```python
from build123d import *

# Parameters (mm, degrees)
F0_W      = 50.8
F0_H      = 50.8
F1_DEPTH  = 50.8
F2_R      = 9
F3_DEPTH  = 407.416
F4_W      = 60.1204171121
F4_H      = 25.4
F5_DEPTH  = 338.582
F6_R      = 5.08
F7_DEPTH  = 5.08
F8_R      = 2.159
F9_DEPTH  = 25.4
F10_R     = 1.5494
F11_DEPTH = 25.4
F12_R     = 1.5494
F12_R_2   = 2.159
F13_DEPTH = 25.4
F14_R     = 5.08
F15_DEPTH = 5.08
F19_DEPTH = 72.39
F22_R     = 12.7


with BuildPart() as f1:
    # F0 (on Top) → F1 (new body)
    with BuildSketch(Plane.XY):
        Rectangle(F0_W, F0_H)
    extrude(amount=F1_DEPTH)

    # F2 (on face) → F3 (cut)
    with BuildSketch(Plane(origin=(0, 0, 0), x_dir=(1, 0, 0), z_dir=(0, 0, -1))):
        Circle(F2_R)
    extrude(amount=-F3_DEPTH, mode=Mode.SUBTRACT)

    # F4 (on face) → F5 (cut)
    with BuildSketch(Plane(origin=(0, 0, 0), x_dir=(1, 0, 0), z_dir=(0, 0, -1))):
        with Locations((4.6602085561, 12.7)):
            Rectangle(F4_W, F4_H)
    extrude(amount=-F5_DEPTH, mode=Mode.SUBTRACT)

    # F6 (on face) → F7 (cut)
    with BuildSketch(Plane.XZ):
        with Locations((-17.2, 25.4)):
            Circle(F6_R)
    extrude(amount=-F7_DEPTH, mode=Mode.SUBTRACT)

    # F8 (on face) → F9 (cut)
    with BuildSketch(Plane.XZ.offset(-5.08)):
        with Locations((-17.2, 25.4)):
            Circle(F8_R)
    extrude(amount=-F9_DEPTH, mode=Mode.SUBTRACT)

    # F10 (on face) → F11 (cut)
    with BuildSketch(Plane.XZ):
        with Locations((-17.2, 44.4713309407)):
            Circle(F10_R)
    extrude(amount=-F11_DEPTH, mode=Mode.SUBTRACT)

    # F12 (on face) → F13 (cut)
    with BuildSketch(Plane.XZ):
        with Locations((17.2, 44.4713309407)):
            Circle(F12_R)
        with Locations((17.2, 25.4)):
            Circle(F12_R_2)
    extrude(amount=-F13_DEPTH, mode=Mode.SUBTRACT)

    # F14 (on face) → F15 (cut)
    with BuildSketch(Plane.XZ):
        with Locations((17.2, 25.4)):
            Circle(F14_R)
    extrude(amount=-F15_DEPTH, mode=Mode.SUBTRACT)

    # F17: F1 across plane


with BuildPart() as f1_1:
    add(f1.part)
    add(f1.part.mirror(Plane(origin=(0, 13.6714489466, 25.4), x_dir=(1, 0, 0), z_dir=(0, 0, 1))), mode=Mode.INTERSECT)

    # F18 (on face) → F19 (cut)
    with BuildSketch(Plane(origin=(0, 0, 0), x_dir=(1, 0, 0), z_dir=(0, 0, -1))):
        Polygon((37.3146161437, -15.35), (0, -15.35), (-44.7141490877, -15.35), (-42.6479764283, -31.9298505783), (43.3826521039, -33.9571945369), align=None)
    extrude(amount=-F19_DEPTH, mode=Mode.SUBTRACT)

    # F22
    f22_edges = [f1_1.edges().sort_by_distance(p)[0] for p in [
        (25.4, 7.675, 50.8),
        (25.4, 7.675, 0),
        (-25.4, 7.675, 50.8),
        (-25.4, 7.675, 0),
    ]]
    fillet(f22_edges, radius=F22_R)


solid = f1_1.part
```
The model under review builds one solid part; all positions refer to its coordinate system, in mm. A direction names the side the tool comes from. Give positions to 0.01 mm unless a question says otherwise; leave off trailing zeros. Write each loop counter-clockwise with the first axis right and the second up, starting at its lowest first coordinate (ties: lowest second). Pieces come first, ordered by that corner, then holes. Notation, with made-up numbers: M 7.5,68 L 61.5,68 A11 cw 61.5,87 Z; hole C 4.5,58.25 d2. An arc over 180 degrees is marked long. Write each question's results on one line, items separated by ' | '. Start each with the question number.
1. We need section B-B (z = 25.4). Write out the cut boundary in (x, y).
2. Insertion check: pin 1 Ø5.5 at (x, z) = (-17.2, 25.4) entering from -Y; pin 2 Ø3 at (x, y) = (18, 11) entering from +Z; pin 3 Ø1.9 at (x, z) = (17.2, 44.47) entering from -Y. Each pin has a flat end and moves straight along its axis. Give the tip position at first contact, or say it passes through.
3. For probe 1 along Z at (x, y) = (-17.2, 3.95); probe 2 along Z at (x, y) = (-17.2, 8.75); probe 3 along X at (y, z) = (12.25, 44), list the stretches that pass through material, from the lowest coordinate up. Write a range as [from, to].
4. Mouldability with a two-part tool opening along X and no side actions: class faces 1 (the flat face through (25.4, 8, 25)), 2 (the cylindrical face through (16.86, 7.57, 7.84)), 3 (the flat face through (-0.2, 9.5, 0)) as released by +X, released by -X, zero draft, split by the parting line, or undercut.
5. We need section C-C (x = 17.2). Write out the cut boundary in (y, z), and give its area (3 significant figures).
6. For faces 4 (the cylindrical face through (0, 9, 25)), 5 (the cylindrical face through (-20.944, 2.504, 28.833)), list the 3-axis set-ups (+Z, -Z, +X, -X, +Y, -Y) from which the entire face can be reached by the end or side of a thin tool; tool diameter is ignored.
7. We need section A-A (y = 7.75). Write out the cut boundary in (x, z).
8. We need section D-D (y = 11.5). Write out the cut boundary in (x, z).
Results found:
1) outline: M -25.4,0 L -22.28,0 L -22.28,5.08 L -19.36,5.08 L -19.36,15.35 L -25.4,15.35 Z; M -15.04,5.08 L -12.12,5.08 L -12.12,0 L -9,0 A9 cw 9,0 L 12.12,0 L 12.12,5.08 L 15.04,5.08 L 15.04,15.35 L -15.04,15.35 Z; M 19.36,5.08 L 22.28,5.08 L 22.28,0 L 25.4,0 L 25.4,15.35 L 19.36,15.35 Z
2) pin 1: stops at y = 5.08 | pin 2: stops at z = 50.22 | pin 3: passes through
3) probe 1: z = [0.82, 4.78], [7.88, 20.32], [30.48, 42.92], [46.02, 49.98] | probe 2: z = [0.82, 4.78], [7.88, 23.24], [27.56, 42.92], [46.02, 49.98] | probe 3: x = [-23.95, -18.68], [-15.72, 15.72], [18.68, 23.95]
4) face 1: released by +X | face 2: undercut | face 3: zero draft
5) outline: M 0,0.82 L 15.35,0.82 L 15.35,4.78 L 0,4.78 Z; M 0,7.88 L 15.35,7.88 L 15.35,23.24 L 5.08,23.24 L 5.08,20.32 L 0,20.32 Z; M 0,30.48 L 5.08,30.48 L 5.08,27.56 L 15.35,27.56 L 15.35,42.92 L 0,42.92 Z; M 0,46.02 L 15.35,46.02 L 15.35,49.98 L 0,49.98 Z | area: 563 mm^2
6) face 4: +Z, -Z, -Y | face 5: -Y
7) outline: M -25.4,12.7 A12.7 ccw -12.7,0 L -4.58,0 L -4.58,50.8 L -12.7,50.8 A12.7 ccw -25.4,38.1 Z; M 4.58,0 L 12.7,0 A12.7 ccw 25.4,12.7 L 25.4,38.1 A12.7 ccw 12.7,50.8 L 4.58,50.8 Z; hole C -17.2,25.4 d4.32; hole C -17.2,6.33 d3.1; hole C -17.2,44.47 d3.1; hole C 17.2,25.4 d4.32; hole C 17.2,6.33 d3.1; hole C 17.2,44.47 d3.1
8) outline: M -25.4,12.7 A12.7 ccw -12.7,0 L 12.7,0 A12.7 ccw 25.4,12.7 L 25.4,38.1 A12.7 ccw 12.7,50.8 L -12.7,50.8 A12.7 ccw -25.4,38.1 Z; hole C -17.2,25.4 d4.32; hole C -17.2,6.33 d3.1; hole C -17.2,44.47 d3.1; hole C 17.2,25.4 d4.32; hole C 17.2,6.33 d3.1; hole C 17.2,44.47 d3.1
